Geometry check sheet. Reference: the model listing, model coordinates, mm. Face numbers are marked on the shaded views. A direction names the side the tool comes from. Round coordinates to 2 decimals unless told otherwise and drop trailing zeros. Order: outer loops, then holes, each group sorted by start corner. A loop starts at its lowest first (then second) coordinate and runs counter-clockwise, first axis right, second up.
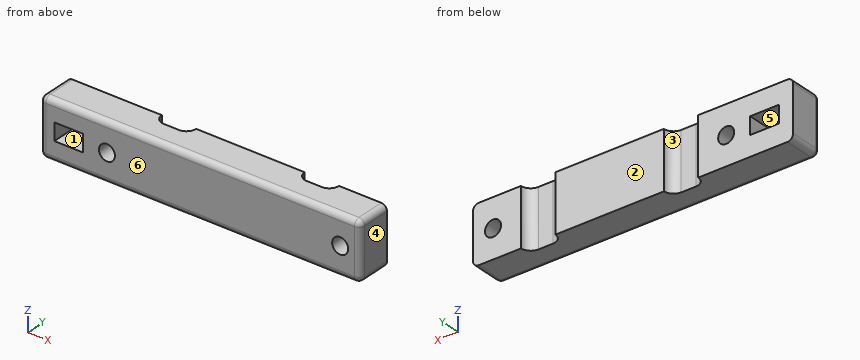
```python
from build123d import *

# Parameters (mm, degrees)
SKETCH1_W                 = 56
SKETCH1_H                 = 10
SKETCH1_R                 = 1.4
SKETCH1_W_2               = 5
SKETCH1_H_2               = 3
BASE_DEPTH                = 6
BASKET_WIRE_GROOVES_DEPTH = 31.331501776
F_1MM_EDGE_FILLETS_R      = 1


with BuildPart() as part:
    # Sketch1 → Base (new body)
    with BuildSketch(Plane(origin=(0, 0, 0), x_dir=(1, 0, 0), z_dir=(0, 1, 0))):
        Rectangle(SKETCH1_W, SKETCH1_H)
        with Locations(Location((-16.3, 0, 0), (0, 0, 270))):
            Circle(SKETCH1_R, mode=Mode.SUBTRACT)
        with Locations(Location((24.5, 0, 0), (0, 0, 270))):
            Circle(SKETCH1_R, mode=Mode.SUBTRACT)
        with Locations((-23, 0)):
            Rectangle(SKETCH1_W_2, SKETCH1_H_2, mode=Mode.SUBTRACT)
    extrude(amount=BASE_DEPTH)

    # Sketch2 → Basket Wire Grooves (cut, through all)
    with BuildSketch(Plane(origin=(0, 0, -5), x_dir=(-1, 0, 0), z_dir=(0, 0, -1))):
        with BuildLine():
            Line((-13.6, 6), (-19.6, 6))
            ThreePointArc((-19.6, 6), (-19.102081528, 4.797918472), (-17.9, 4.3))
            Line((-17.9, 4.3), (-15.3, 4.3))
            ThreePointArc((-15.3, 4.3), (-14.097918472, 4.797918472), (-13.6, 6))
        make_face()
        with BuildLine():
            Line((5.4, 6), (11.4, 6))
            ThreePointArc((11.4, 6), (10.902081528, 4.797918472), (9.7, 4.3))
            Line((9.7, 4.3), (7.1, 4.3))
            ThreePointArc((7.1, 4.3), (5.897918472, 4.797918472), (5.4, 6))
        make_face()
    extrude(amount=-BASKET_WIRE_GROOVES_DEPTH, mode=Mode.SUBTRACT)

    # 1mm Edge Fillets
    f_1mm_edge_fillets_edges = [part.edges().sort_by_distance(p)[0] for p in [
        (0, 0, 5),
        (-28, 0, 0),
        (0, 0, -5),
        (28, 0, 0),
        (28, 3, 5),
        (-28, 3, 5),
        (-28, 3, -5),
        (28, 3, -5),
    ]]
    fillet(f_1mm_edge_fillets_edges, radius=F_1MM_EDGE_FILLETS_R)


solid = part.part
```
(1) Set-up check for the marked faces 1, 2 and 3: record each of +Z, -Z, +X, -X, +Y, -Y from which the full face is reachable in a straight line by a thin tool's end or side.
Returned:
face 1: +Y, -Y
face 2: +Z, -Z, +X, -X, +Y
face 3: +Z, -Z, +Y
(2) Draft check along X on the marked faces 4, 5 and 6. Enter one of: released by +X, released by -X, zero draft, split by the parting line, or undercut.
Returned:
face 4: released by +X
face 5: undercut
face 6: zero draft
(3) Sectioned sample at C-C, the plane y = 1.7. Record the cut outline in (x, z).
Returned:
outline: (-28, -4) arc R1 ccw to (-27, -5) - (27, -5) arc R1 ccw to (28, -4) - (28, 4) arc R1 ccw to (27, 5) - (-27, 5) arc R1 ccw to (-28, 4) - close; hole (-25.5, -1.5) - (-20.5, -1.5) - (-20.5, 1.5) - (-25.5, 1.5) - close; hole circle Ø2.8 at (-16.3, 0); hole circle Ø2.8 at (24.5, 0)
(4) Material ranges on line 1 (X direction, y = 2.6, z = 0); line 2 (X direction, y = 4.9, z = 0); line 3 (Y direction, x = 16, z = -3.75), recorded low to high.
Returned:
line 1: x = -28 to -25.5, -20.5 to -17.7, -14.9 to 23.1, 25.9 to 28
line 2: x = -28 to -25.5, -20.5 to -17.7, -14.9 to -11, -5.8 to 14, 19.2 to 23.1, 25.9 to 28
line 3: y = 0 to 4.3
(5) Depth check by flat-ended pin: P1, Ø2, axis at x = -8, z = -1.5, coming from the +Y side; P2, Ø2, axis at x = -16.3, z = 0, coming from the -Y side. Enter the tip coordinate at first touch or a pass-through.
Returned:
P1: stops at y = 4.3
P2: passes through
(6) Sectioned sample at B-B, the plane z = 0. Record the cut outline in (x, y), and give its area (3 significant figures).
Returned:
outline: (-28, 1) arc R1 ccw to (-27, 0) - (-25.5, 0) - (-25.5, 6) - (-28, 6) - close; (-20.5, 0) - (-17.7, 0) - (-17.7, 6) - (-20.5, 6) - close; (-14.9, 0) - (23.1, 0) - (23.1, 6) - (19.6, 6) arc R1.7 cw to (17.9, 4.3) - (15.3, 4.3) arc R1.7 cw to (13.6, 6) - (-5.4, 6) arc R1.7 cw to (-7.1, 4.3) - (-9.7, 4.3) arc R1.7 cw to (-11.4, 6) - (-14.9, 6) - close; (25.9, 0) - (27, 0) arc R1 ccw to (28, 1) - (28, 6) - (25.9, 6) - close
area: 254 mm2
(7) Sectioned sample at A-A, the plane y = 5.2. Record the cut outline in (x, z).
Returned:
outline: (-28, -4) arc R1 ccw to (-27, -5) - (-11.2, -5) - (-11.2, 5) - (-27, 5) arc R1 ccw to (-28, 4) - close; (-5.6, -5) - (13.8, -5) - (13.8, 5) - (-5.6, 5) - close; (19.4, -5) - (27, -5) arc R1 ccw to (28, -4) - (28, 4) arc R1 ccw to (27, 5) - (19.4, 5) - close; hole (-25.5, -1.5) - (-20.5, -1.5) - (-20.5, 1.5) - (-25.5, 1.5) - close; hole circle Ø2.8 at (-16.3, 0); hole circle Ø2.8 at (24.5, 0)
(8) Sectioned sample at D-D, the plane x = -16.3. Record the cut outline in (y, z).
Returned:
outline: (0, -4) arc R1 ccw to (1, -5) - (6, -5) - (6, -1.4) - (0, -1.4) - close; (0, 1.4) - (6, 1.4) - (6, 5) - (1, 5) arc R1 ccw to (0, 4) - close
